```python
from build123d import *

# Parameters (mm, degrees)
SKETCH1_R               = 7.5
BOSS_EXTRUDE1_DEPTH     = 38
SKETCH2_W               = 23.956439237
SKETCH2_H               = 10
CUT_EXTRUDE1_DEPTH      = 8.5
CUT_EXTRUDE1_DEPTH_BACK = 18.5
FILLET1_R               = 3
FILLET2_R               = 5


with BuildPart() as part:
    # Sketch1 → Boss-Extrude1 (new body)
    with BuildSketch(Plane.XY):
        with BuildLine():
            Line((183.043560763, 5), (11.456439237, 5))
            ThreePointArc((11.456439237, 5), (-12.5, 0), (11.456439237, -5))
            Line((11.456439237, -5), (183.043560763, -5))
            ThreePointArc((183.043560763, -5), (207, 0), (183.043560763, 5))
        make_face()
        Circle(SKETCH1_R, mode=Mode.SUBTRACT)
        with Locations((194.5, 0)):
            Circle(SKETCH1_R, mode=Mode.SUBTRACT)
    extrude(amount=BOSS_EXTRUDE1_DEPTH)

    # Sketch2 → Cut-Extrude1 (cut, two sides)
    with BuildSketch(Plane(origin=(0, 5, 0), x_dir=(1, 0, 0), z_dir=(0, 1, 0))) as cut_extrude1_sk:
        Polygon((11.456439237, -27.558152076), (11.456439237, -28), (11.456439237, -38), (183.043560763, -38), (183.043560763, -35.049807592), align=None)
        with Locations((-0.521780381, -33)):
            Rectangle(SKETCH2_W, SKETCH2_H)
        with Locations((-0.521780381, -5)):
            Rectangle(SKETCH2_W, SKETCH2_H)
        Polygon((183.043560763, 0), (11.456439237, 0), (11.456439237, -10), (11.456439237, -10.441847924), (183.043560763, -2.950192408), align=None)
        Polygon((74.351780381, -15.703399507), (74.351780381, -22.296600493), (174.351780381, -26.662694784), (174.351780381, -11.337305216), align=None)
    extrude(amount=CUT_EXTRUDE1_DEPTH, mode=Mode.SUBTRACT)
    extrude(cut_extrude1_sk.sketch, amount=-CUT_EXTRUDE1_DEPTH_BACK, mode=Mode.SUBTRACT)

    # Fillet1
    fillet1_edges = [part.edges().sort_by_distance(p)[0] for p in [
        (74.351780381, 0, 22.296600493),
        (74.351780381, 0, 15.703399507),
    ]]
    fillet(fillet1_edges, radius=FILLET1_R)

    # Fillet2
    fillet2_edges = [part.edges().sort_by_distance(p)[0] for p in [
        (174.351780381, 0, 11.337305216),
        (174.351780381, 0, 26.662694784),
    ]]
    fillet(fillet2_edges, radius=FILLET2_R)


solid = part.part
```
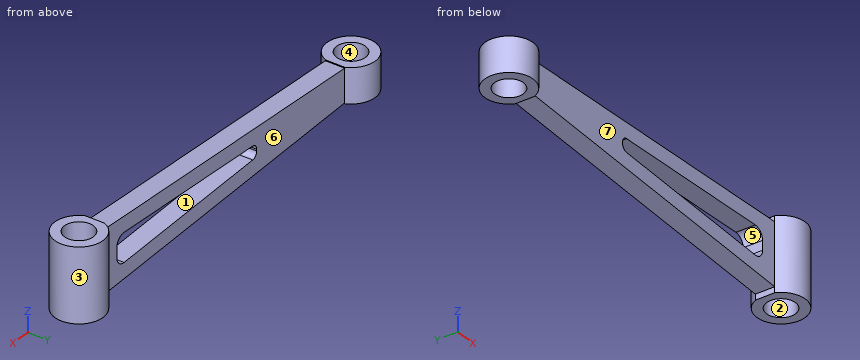
For this review, take the finished solid that the model builds, in its own axes (mm). Face numbers are marked on the shaded views. A direction names the side the tool comes from. Coordinates: 2 decimals unless noted, no trailing zeros. Order: outer loops, then holes, each group sorted by start corner. A loop starts at its lowest first (then second) coordinate and runs counter-clockwise, first axis right, second up. Notation, with made-up numbers: (-19.5, -25.75) -> (35.5, -25.75) arc R10 cw to (35.5, -11.75) -> close; hole circle Ø8 at (78, -27). An arc over 180 degrees is marked (long way). Answer as CSV lines item,"result".
Q1. We need section B-B (x = 194.5). State the section outline as (y, z) points.
Model answer:
outline,"(-12.5, 0) -> (-7.5, 0) -> (-7.5, 38) -> (-12.5, 38) -> close; (7.5, 0) -> (12.5, 0) -> (12.5, 38) -> (7.5, 38) -> close"
Q2. For the marked faces 4, 5, 6 and 7, list the 3-axis set-ups (+Z, -Z, +X, -X, +Y, -Y) from which the entire face can be reached by the end or side of a thin tool; tool diameter is ignored.
Model answer:
face 4,"+Z, -Z"
face 5,"+Y, -Y"
face 6,"+Z, -Z, +Y"
face 7,"+Z, -Z, -Y"
Q3. We need section C-C (y = -10.25). State the section outline as (x, z) points, plus the area to 3 significant figures.
Model answer:
outline,"(-7.15, 10) -> (7.15, 10) -> (7.15, 28) -> (-7.15, 28) -> close; (187.35, 0) -> (201.65, 0) -> (201.65, 38) -> (187.35, 38) -> close"
area,"801 mm2"
Q4. Clearance check with flat-ended pins moving along their axes: pin 1 Ø5 at (y, z) = (3, 8.5) entering from -X; pin 2 Ø2 at (x, y) = (21.5, -3) entering from -Z; pin 3 Ø0.9 at (y, z) = (-1.5, 37) entering from -X. State where each tip first meets the part, or that it passes through.
Model answer:
pin 1,"stops at x = -12.46"
pin 2,"stops at z = 9.96"
pin 3,"stops at x = 183.04"
Q5. We need section D-D (z = 32.5). State the section outline as (x, y) points.
Model answer:
outline,"(124.64, -5) -> (183.04, -5) arc R12.5 ccw (long way) to (183.04, 5) -> (124.64, 5) -> close; hole circle Ø15 at (194.5, 0)"
Q6. Draft analysis for pull direction Y (two halves, no side actions). For the marked faces 1, 2 and 3, state which applies: released by +Y, released by -Y, zero draft, split by the parting line, or undercut.
Model answer:
face 1,"zero draft"
face 2,"undercut"
face 3,"split by the parting line"
Q7. Wall thickness on line 1 along Y through (x, z) = (0, 15.25); line 2 along Z through (x, y) = (-2, 8.75); line 3 along X through (y, z) = (5.5, 13.5): over which ranges is each line inside the solid? List them lowest first. Write a range as [from, to].
Model answer:
line 1,"y = [-12.5, -7.5], [7.5, 12.5]"
line 2,"z = [10, 28]"
line 3,"x = [-11.22, -5.1], [5.1, 11.22], [183.28, 189.4], [199.6, 205.72]"
Q8. We need section A-A (y = 0). State the section outline as (x, z) points.
Model answer:
outline,"(-12.5, 10) -> (-7.5, 10) -> (-7.5, 28) -> (-12.5, 28) -> close; (7.5, 10) -> (11.46, 10) -> (11.46, 10.44) -> (183.04, 2.95) -> (183.04, 0) -> (187, 0) -> (187, 38) -> (183.04, 38) -> (183.04, 35.05) -> (11.46, 27.56) -> (11.46, 28) -> (7.5, 28) -> close; (202, 0) -> (207, 0) -> (207, 38) -> (202, 38) -> close; hole (74.35, 18.58) arc R3 ccw to (77.22, 15.58) -> (169.13, 11.57) arc R5 ccw to (174.35, 16.56) -> (174.35, 21.44) arc R5 ccw to (169.13, 26.43) -> (77.22, 22.42) arc R3 ccw to (74.35, 19.42) -> close"
